Verification items for the finished model (mm, model axes). A direction names the side the tool comes from. Coordinates: 2 decimals unless noted, no trailing zeros. Write each loop counter-clockwise with the first axis right and the second up, starting at its lowest first coordinate (ties: lowest second). Pieces come first, ordered by that corner, then holes.
Autodesk Inventor part; units mm, degrees
ref_plane "YZ Plane" through (0, 0, 0) normal (1, 0, 0) x (0, 1, 0)
ref_plane "XZ Plane" through (0, 0, 0) normal (0, 1, 0) x (-1, 0, 0)
ref_plane "XY Plane" through (0, 0, 0) normal (0, 0, 1) x (1, 0, 0)
sketch "Sketch1" plane through (0, 0, 0) normal (1, 0, 0) x (0, 1, 0)
  line L0 (9.8886, 10.374) -> (-32.1114, 10.374)
  line L1 (-32.1114, 10.374) -> (-32.1114, -37.736)
  line L2 (-32.1114, -37.736) -> (9.8886, -37.736)
  line L3 (9.8886, -37.736) -> (9.8886, 10.374)
  point P0 (0, 0)
  dimension "d0" = 42
  dimension "d1" = 48.11
extrude "Extrusion1" add sketch "Sketch1" along normal blind 3
sketch "Sketch2" plane through (3, 0, 0) normal (1, 0, 0) x (0, 0, -1)
  line L0 (-7.974, 7.4886) -> (35.336, 7.4886)
  line L1 (35.336, 7.4886) -> (35.336, -30.1114)
  line L2 (35.336, -30.1114) -> (-7.974, -30.1114)
  line L3 (-7.974, -30.1114) -> (-7.974, 7.4886)
  line L4 (37.736, 9.8886) -> (-10.374, 9.8886)
  line L5 (-10.374, 9.8886) -> (-10.374, -32.1114)
  line L6 (-10.374, -32.1114) -> (37.736, -32.1114)
  point P0 (0, 0)
  dimension "d4" = 43.31
  dimension "d6" = 2.4
  dimension "d7" = 2.4
  dimension "d20" = 2
extrude "Extrusion2" add sketch "Sketch2" along normal blind 3
sketch "Sketch3" plane through (3, 0, 0) normal (1, 0, 0) x (0, 0, -1)
  line L0 (-10.374, 9.8886) -> (-10.374, -32.1114)
  line L1 (-7.974, -30.1114) -> (-7.974, 7.4886)
  line L2 (-10.374, -29.3114) -> (-7.974, -29.3114)
  line L3 (-7.974, -29.3114) -> (-7.974, -17.1114)
  line L4 (-7.974, -17.1114) -> (-10.374, -17.1114)
  line L5 (-10.374, -17.1114) -> (-10.374, -29.3114)
  line L6 (-10.374, -32.1114) -> (37.736, -32.1114)
  point P0 (0, 0)
  point P1 (-10.374, 9.3886)
  point P2 (-10.374, -31.6114)
  point P3 (-7.974, -29.6114)
  point P4 (-7.974, 6.9886)
  point P5 (-9.874, -32.1114)
  point P6 (37.236, -32.1114)
  point P7 (-7.974, -29.3114)
  dimension "d12" = 12.2
  dimension "d13" = 2.8
extrude "PowerSocket" add sketch "Sketch3" along normal blind 6.6
sketch "Sketch5" plane through (3, 0, 0) normal (1, 0, 0) x (0, 0, -1)
  line L0 (-10.374, 9.8886) -> (-10.374, -17.1114)
  line L1 (-7.974, -17.1114) -> (-7.974, 7.4886)
  line L2 (-10.374, -6.6114) -> (-7.974, -6.6114)
  line L3 (-7.974, -6.6114) -> (-7.974, 6.7886)
  line L4 (-7.974, 6.7886) -> (-10.374, 6.7886)
  line L5 (-10.374, 6.7886) -> (-10.374, -6.6114)
  line L6 (-7.974, -17.1114) -> (-10.374, -17.1114)
  line L7 (35.336, 7.4886) -> (-7.974, 7.4886)
  line L8 (37.736, 9.8886) -> (-10.374, 9.8886)
  point P0 (0, 0)
  point P1 (-10.374, 9.3886)
  point P2 (-10.374, 6.7886)
  point P3 (-7.974, -6.6114)
  point P4 (37.236, 9.8886)
  point P5 (-9.874, 9.8886)
  dimension "d21" = 13.4
  dimension "d75" = 3.1
extrude "RJ-12" add sketch "Sketch5" along normal blind 6.6 contours L4 L1 L2 L0
sketch "Sketch6" plane through (3, 0, 0) normal (1, 0, 0) x (0, 0, -1)
  line L0 (-10.374, -32.1114) -> (37.736, -32.1114)
  line L1 (-7.974, -30.1114) -> (35.336, -30.1114)
  line L2 (12.726, -32.1114) -> (3.526, -32.1114)
  line L3 (3.526, -32.1114) -> (3.526, -30.1114)
  line L4 (3.526, -30.1114) -> (12.726, -30.1114)
  line L5 (12.726, -30.1114) -> (12.726, -32.1114)
  line L6 (-10.374, -29.3114) -> (-10.374, -32.1114)
  point P0 (0, 0)
  point P1 (-9.874, -32.1114)
  point P2 (37.236, -32.1114)
  point P3 (-10.374, -31.6114)
  dimension "d25" = 9.2
  dimension "d26" = 13.9
extrude "USB-C" add sketch "Sketch6" along normal blind 6.6
sketch "Sketch7" plane through (6, 0, 0) normal (1, 0, 0) x (0, 0, -1)
  line L0 (35.336, 7.4886) -> (-7.974, 7.4886)
  line L1 (-7.974, 7.4886) -> (-5.974, 7.4886)
  line L2 (-5.974, 7.4886) -> (-5.974, -30.1114)
  line L3 (-7.974, -30.1114) -> (3.526, -30.1114)
  line L4 (-5.974, -30.1114) -> (-7.974, -30.1114)
  line L5 (-10.374, -29.3114) -> (-10.374, -32.1114)
  line L6 (-7.974, 7.4886) -> (-7.974, -17.1114)
  line L7 (-7.974, -30.1114) -> (-7.974, 7.4886)
  line L8 (35.336, -30.1114) -> (12.726, -30.1114)
  line L9 (-5.974, -30.1114) -> (35.336, -30.1114)
  line L10 (35.336, -30.1114) -> (35.336, -28.1114)
  line L11 (35.336, 7.4886) -> (35.336, -30.1114)
  line L12 (35.336, -28.1114) -> (-5.974, -28.1114)
  line L13 (35.336, -28.1114) -> (35.336, 7.4886)
  line L14 (35.336, 7.4886) -> (33.336, 7.4886)
  line L15 (33.336, 7.4886) -> (33.336, -28.1114)
  line L16 (33.336, 7.4886) -> (3.336, 7.4886)
  line L17 (3.336, 7.4886) -> (3.336, 5.4886)
  line L18 (3.336, 5.4886) -> (33.336, 5.4886)
  point P0 (0, 0)
  point P1 (-10.374, -31.6114)
  point P2 (-7.974, 6.7886)
  point P3 (-7.974, 6.6886)
  dimension "d29" = 2
  dimension "d30" = 2
  dimension "d31" = 2
  dimension "d32" = 2
  dimension "d33" = 30
  dimension "d34" = 2
extrude "Extrusion7" add sketch "Sketch7" along normal blind 2 contours L11 L12 L15 L0 | L15 L18 L17 L0 | L10 L8 L9 L3 L2 L12 | L2 L3 L7 L6 L0
sketch "Sketch8" plane through (3, -30.1114, -3.526) normal (0, -1, 0) x (1, 0, 0)
  line L0 (2, 8.5) -> (1, 8.5)
  line L1 (1, 8.5) -> (1, 3.5)
  line L2 (1, 3.5) -> (2, 3.5)
  line L3 (2, 3.5) -> (2, 8.5)
  line L4 (0, 11.5) -> (5, 11.5)
  line L5 (5, 11.5) -> (5, 0)
  line L6 (0, 13.9) -> (0, 0)
  point P0 (-3, 3.526)
  point P1 (2, 6)
  point P2 (0, 13.4)
  dimension "d37" = 1
  dimension "d38" = 5
  dimension "d39" = 5.5
  dimension "d60" = 1
extrude "Extrusion8" add sketch "Sketch8" along normal blind 0.5
fillet "Fillet3" radius 0.5 4 edges at (5, -30.6114, 2.474) (4, -30.6114, 2.474) (4.5, -30.6114, 4.974) (4.5, -30.6114, -0.026)
sketch "Sketch9" plane through (3, -30.1114, -35.336) normal (0, -1, 0) x (1, 0, 0)
  line L0 (2, 13.5) -> (1, 13.5)
  line L1 (1, 13.5) -> (1, 8.5)
  line L2 (1, 8.5) -> (2, 8.5)
  line L3 (2, 8.5) -> (2, 13.5)
  line L4 (5, 22.61) -> (5, 0)
  line L5 (0, 0) -> (5, 0)
  line L6 (0, 22.61) -> (0, -2.4)
  point P0 (-3, 35.336)
  point P1 (2, 11)
  point P2 (0, -1.9)
  dimension "d44" = 1
  dimension "d45" = 5
  dimension "d47" = 11
  dimension "d59" = 1
extrude "Extrusion9" add sketch "Sketch9" along normal blind 0.5
fillet "Fillet4" radius 0.5 4 edges at (5, -30.6114, -24.336) (4, -30.6114, -24.336) (4.5, -30.6114, -21.836) (4.5, -30.6114, -26.836)
sketch "Sketch10" plane through (3, 7.4886, 7.974) normal (0, 1, 0) x (1, 0, 0)
  line L0 (2, 34.81) -> (1, 34.81)
  line L1 (1, 34.81) -> (1, 29.81)
  line L2 (1, 29.81) -> (2, 29.81)
  line L3 (2, 29.81) -> (2, 34.81)
  line L4 (5, 43.31) -> (5, 11.31)
  line L5 (0, 43.31) -> (5, 43.31)
  line L6 (0, 45.71) -> (0, -2.4)
  point P0 (-3, 7.974)
  point P1 (2, 32.31)
  point P2 (0, 45.21)
  point P3 (0, -1.9)
  dimension "d51" = 1
  dimension "d52" = 5
  dimension "d54" = 11
  dimension "d58" = 1
extrude "Extrusion10" add sketch "Sketch10" along normal blind 0.5
fillet "Fillet5" radius 0.5 4 edges at (5, 7.9886, -24.336) (4, 7.9886, -24.336) (4.5, 7.9886, -26.836) (4.5, 7.9886, -21.836)
sketch "Sketch11" plane through (3, 7.4886, 7.974) normal (0, 1, 0) x (1, 0, 0)
  line L0 (2, 8) -> (1, 8)
  line L1 (1, 8) -> (1, 3)
  line L2 (1, 3) -> (2, 3)
  line L3 (2, 3) -> (2, 8)
  line L4 (0, 45.71) -> (0, -2.4)
  line L5 (0, 0) -> (5, 0)
  point P0 (-3, 7.974)
  point P1 (0, 45.21)
  point P2 (0, -1.9)
  point P3 (1, 5.5)
  dimension "d61" = 1
  dimension "d62" = 5
  dimension "d63" = 1
  dimension "d64" = 5.5
extrude "Extrusion11" add sketch "Sketch11" along normal blind 0.5
fillet "Fillet6" radius 0.5 4 edges at (5, 7.9886, 2.474) (4, 7.9886, 2.474) (4.5, 7.9886, 4.974) (4.5, 7.9886, -0.026)
fillet "Fillet7" radius 0.5 4 edges at (5.5, -30.1114, -35.336) (5.5, 7.4886, -35.336) (5.5, 7.4886, 7.974) (5.5, -30.1114, 7.974)
sketch "Sketch14" plane through (0, -32.1114, -37.736) normal (0, -1, 0) x (1, 0, 0)
  line L0 (12.0388, 48.7944) -> (-2.0784, 48.7944)
  line L1 (-2.0784, 48.7944) -> (-2.0784, -2.1843)
  line L2 (-2.0784, -2.1843) -> (12.0388, -2.1843)
  line L3 (12.0388, -2.1843) -> (12.0388, 48.7944)
  point P0 (0, 37.736)
extrude "TrimmWall" cut sketch "Sketch14" against normal blind 0.83
fillet "Fillet8" radius 0.5 4 edges at (1.5, -31.2814, -37.736) (1.5, 9.8886, -37.736) (1.5, -31.2814, 10.374) (1.5, 9.8886, 10.374)
sketch "Sketch15" plane through (3, 0, 0) normal (1, 0, 0) x (0, 0, -1)
  arc A0 (-4.974, -30.1114) -> (-4.474, -30.6114) centre (-4.474, -30.1114) ccw
  line L0 (-9.874, -31.2814) -> (3.526, -31.2814)
  line L1 (-4.974, -30.1114) -> (0.026, -30.1114)
  line L2 (0.026, -30.1114) -> (0.026, -31.2814)
  line L3 (0.026, -31.2814) -> (-4.974, -31.2814)
  line L4 (-4.974, -31.2814) -> (-4.974, -30.1114)
  arc A1 (21.836, -30.1114) -> (22.336, -30.6114) centre (22.336, -30.1114) ccw
  line L5 (12.726, -31.2814) -> (37.236, -31.2814)
  line L6 (21.836, -30.1114) -> (26.836, -30.1114)
  line L7 (26.836, -30.1114) -> (26.836, -31.2814)
  line L8 (26.836, -31.2814) -> (21.836, -31.2814)
  line L9 (21.836, -31.2814) -> (21.836, -30.1114)
  point P0 (0, 0)
  dimension "d79" = 5
  dimension "d80" = 5
extrude "Oeffnungskerben1" cut sketch "Sketch15" against normal blind 0.25
sketch "Sketch16" plane through (3, 0, 0) normal (1, 0, 0) x (0, 0, -1)
  arc A0 (26.836, 7.4886) -> (26.336, 7.9886) centre (26.336, 7.4886) ccw
  line L0 (37.236, 9.8886) -> (-9.874, 9.8886)
  line L1 (26.836, 7.4886) -> (21.836, 7.4886)
  line L2 (21.836, 7.4886) -> (21.836, 9.8886)
  line L3 (21.836, 9.8886) -> (26.836, 9.8886)
  line L4 (26.836, 9.8886) -> (26.836, 7.4886)
  arc A1 (0.026, 7.4886) -> (-0.474, 7.9886) centre (-0.474, 7.4886) ccw
  line L5 (0.026, 7.4886) -> (-4.974, 7.4886)
  line L6 (-4.974, 7.4886) -> (-4.974, 9.8886)
  line L7 (-4.974, 9.8886) -> (0.026, 9.8886)
  line L8 (0.026, 9.8886) -> (0.026, 7.4886)
  point P0 (0, 0)
  dimension "d83" = 5
  dimension "d84" = 5
extrude "Oeffnungskerben2" cut sketch "Sketch16" against normal blind 0.25
properties part number "Enclosure_Bottom"
1. Draft check along Y on faces 1 (the flat face through (1, 9.889, -14)), 2 (the flat face through (7, 5.489, -18)), 3 (the flat face through (3, 8, 8)). Enter one of: pulls with the +Y half, pulls with the -Y half, needs draft (parallel to the pull), parting line crosses it, or undercut.
2. Sectioned sample at C-C, the plane z = -1.5. Record the boundary of the cut face in (x, y).
3. Tool access check on faces 4 (the flat face through (2.75, 9, 3)), 5 (the flat face through (2.75, -31, -24)), 6 (the flat face through (9, -30.111, -8)), 7 (the flat face through (5, -11, -35.336)). Record the directions out of +Z, -Z, +X, -X, +Y, -Y that give a thin tool (end or side, any length) a straight path to the whole face; none if there is none.
4. Material ranges on L1, parallel to Y at x = 7.75, z = -8.5; L2, parallel to Z at x = 7.75, y = 6.5; L3, parallel to Y at x = 7.5, z = -15, recorded low to high.
5. Sectioned sample at B-B, the plane z = -30. Record the boundary of the cut face in (x, y).
6. Gauge pin test, flat ends, axial feed: P1, Ø5, axis at x = 8, z = -20.5, coming from the -Y side; P2, Ø3.5, axis at y = -17.5, z = -32.5, coming from the +X side; P3, Ø2, axis at y = -3.5, z = -20.5, coming from the +X side. Record the tip position at first contact, or that the pin passes through.
7. Sectioned sample at A-A, the plane y = -12.5. Record the boundary of the cut face in (x, z).
Outcome:
1. face 1: pulls with the +Y half
1. face 2: undercut
1. face 3: needs draft
2. outline: (0, -31.28) - (3, -31.28) - (3, -30.11) - (8, -30.11) - (8, -28.11) - (6, -28.11) - (6, 7.49) - (3, 7.49) - (3, 9.89) - (0, 9.89) - close
3. face 4: +Y
3. face 5: -Y
3. face 6: +Z, -Z, +X, +Y
3. face 7: -Z, +X, +Y, -Y
4. L1: y = -31.28 to -28.11, 5.49 to 7.49
4. L2: z = -35.34 to -3.34, 5.97 to 10.37
4. L3: y = -30.11 to -28.11, 5.49 to 7.49
5. outline: (0, -31.28) - (3, -31.28) - (3, -30.11) - (8, -30.11) - (8, -28.11) - (6, -28.11) - (6, 5.49) - (8, 5.49) - (8, 7.49) - (3, 7.49) - (3, 9.89) - (0, 9.89) - close
6. P1: stops at y = -30.11
6. P2: stops at x = 8
6. P3: stops at x = 6
7. outline: (0, -37.74) - (3, -37.74) - (3, -35.34) - (8, -35.34) - (8, -33.34) - (6, -33.34) - (6, 5.97) - (8, 5.97) - (8, 7.97) - (3, 7.97) - (3, 10.37) - (0, 10.37) - close
